Geometry check sheet. Reference: drawing and pictorial views, mm from the part's lowest x, y, z. Coordinates: 2 decimals unless noted, no trailing zeros. Write each loop counter-clockwise with the first axis right and the second up, starting at its lowest first coordinate (ties: lowest second). Pieces come first, ordered by that corner, then holes. Notation, with made-up numbers: (75, -11) -> (127, -11) arc R28 ccw to (127, 15) -> close; hole circle Ø4 at (18.5, 73). An arc over 180 degrees is marked (long way). Use a Markdown table: item, result. Add a question column.
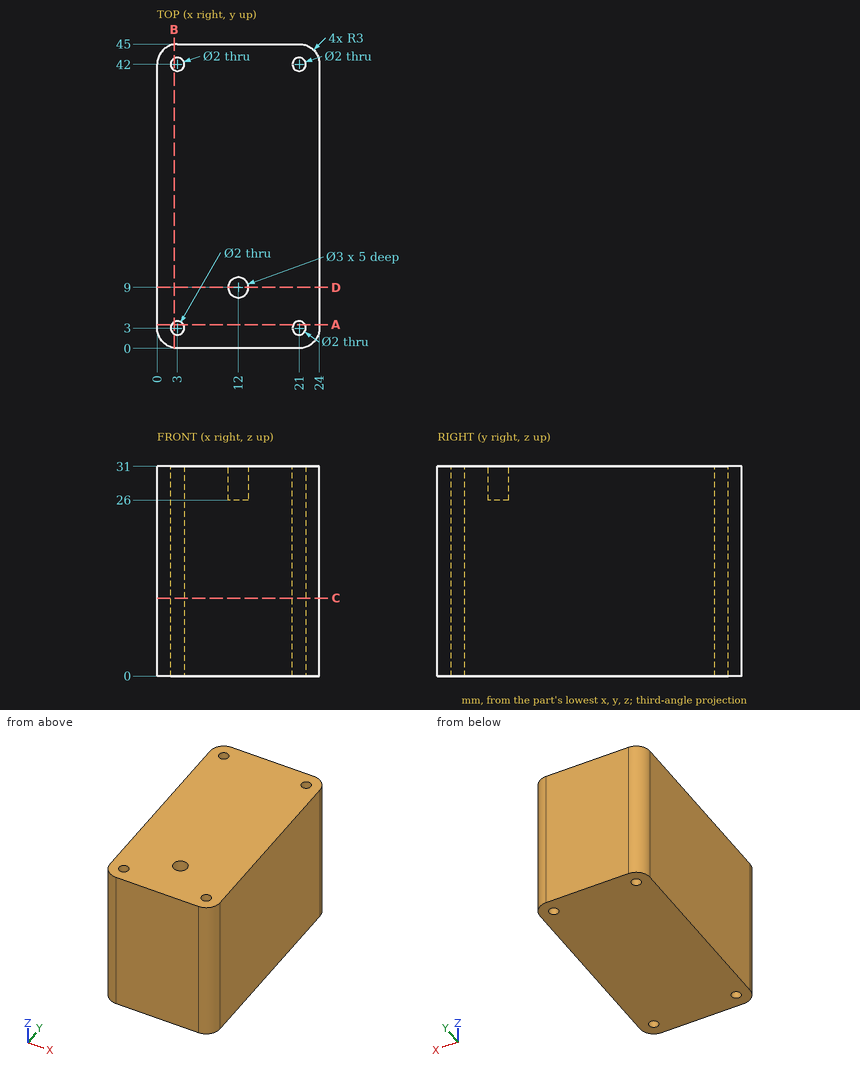
1) Cross-section at A-A on y = 3.5. Record the boundary of the cut face in (x, z), then the cut area to 3 significant figures.
2) Thickness scan on L1, parallel to Y at x = 21, z = 20.5; L2, parallel to X at y = 41.5, z = 28.5; L3, parallel to Y at x = 20.5, z = 5.5. Record the ranges inside material, lowest first.
3) Cross-section at D-D on y = 9. Record the boundary of the cut face in (x, z), then the cut area to 3 significant figures.
4) Cross-section at C-C on z = 11.5. Record the boundary of the cut face in (x, y).
5) Cross-section at B-B on x = 2.5. Record the boundary of the cut face in (y, z), then the cut area to 3 significant figures.
6) Gauge pin test, flat end, axial feed: pin 1 (1.2 mm diameter, centred on x = 21, y = 42, fed in from -Z). Record the tip position at first contact, or that the pin passes through.
Returned:
| question | item | result |
|---|---|---|
| 1 | outline | (0, 0) -> (2.13, 0) -> (2.13, 31) -> (0, 31) -> close; (3.87, 0) -> (20.13, 0) -> (20.13, 31) -> (3.87, 31) -> close; (21.87, 0) -> (24, 0) -> (24, 31) -> (21.87, 31) -> close |
| 1 | area | 637 mm² |
| 2 | L1 | y = 0 to 2, 4 to 41, 43 to 45 |
| 2 | L2 | x = 0 to 2.13, 3.87 to 20.13, 21.87 to 24 |
| 2 | L3 | y = 0 to 2.13, 3.87 to 41.13, 42.87 to 45 |
| 3 | outline | (0, 0) -> (24, 0) -> (24, 31) -> (13.5, 31) -> (13.5, 26) -> (10.5, 26) -> (10.5, 31) -> (0, 31) -> close |
| 3 | area | 729 mm² |
| 4 | outline | (0, 3) arc R3 ccw to (3, 0) -> (21, 0) arc R3 ccw to (24, 3) -> (24, 42) arc R3 ccw to (21, 45) -> (3, 45) arc R3 ccw to (0, 42) -> close; hole circle Ø2 at (3, 3); hole circle Ø2 at (3, 42); hole circle Ø2 at (21, 3); hole circle Ø2 at (21, 42) |
| 5 | outline | (0.04, 0) -> (2.13, 0) -> (2.13, 31) -> (0.04, 31) -> close; (3.87, 0) -> (41.13, 0) -> (41.13, 31) -> (3.87, 31) -> close; (42.87, 0) -> (44.96, 0) -> (44.96, 31) -> (42.87, 31) -> close |
| 5 | area | 1,290 mm² |
| 6 | pin 1 | passes through |
